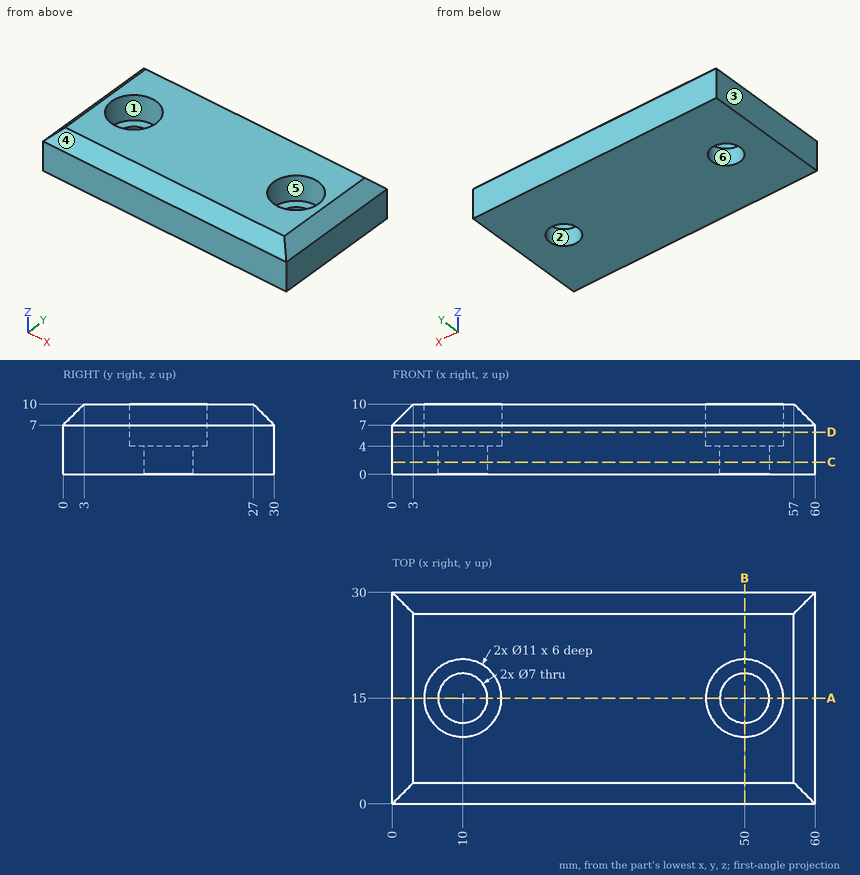
Answer from the drawing. Dimensions are ordinates in mm from the lowest x, y and z of the part. A direction names the side the tool comes from. Round coordinates to 2 decimals unless told otherwise and drop trailing zeros. Order: outer loops, then holes, each group sorted by start corner. A loop starts at its lowest first (then second) coordinate and runs counter-clockwise, first axis right, second up.
1) For the marked faces 5 and 6, determine the directions among +Z, -Z, +X, -X, +Y, -Y from which every point of the face is accessible in a straight line to the end or side of a thin tool.
2) The part is cut by section D-D on z = 6. Write down the section's boundary in (x, y), plus the area to 3 significant figures.
3) The mould has two halves that part along X. Classify the marked faces 1, 2, 3 and 4: released by +X, released by -X, zero draft, split by the parting line, or undercut.
4) Straight lines are drawn through the part: L1, parallel to Y at x = 50, z = 1.1; L2, parallel to X at y = 19, z = 7.5; L3, parallel to X at y = 20, z = 7.25. For each, find the intervals that lie inside material, in ascending order.
5) The part is cut by section B-B on x = 50. Write down the section's boundary in (y, z).
6) Flat-ended cylindrical pins translate along their axes: pin 1 (5.5 mm diameter, centred on x = 50, y = 15, fed in from +Z); pin 2 (1.5 mm diameter, centred on y = 18, z = 8.5, fed in from -X). Find the tip coordinate at first contact, or state that the pin passes through.
7) The part is cut by section A-A on y = 15. Write down the section's boundary in (x, z).
8) The part is cut by section C-C on z = 1.75. Write down the section's boundary in (x, y), plus the area to 3 significant figures.
Resolved:
1. face 5: +Z
1. face 6: +Z, -Z
2. outline: (0, 0) - (60, 0) - (60, 30) - (0, 30) - close; hole circle Ø11 at (10, 15); hole circle Ø11 at (50, 15)
2. area: 1,610 mm2
3. face 1: undercut
3. face 2: undercut
3. face 3: released by -X
3. face 4: zero draft
4. L1: y = 0 to 11.5, 18.5 to 30
4. L2: x = 0.5 to 6.23, 13.77 to 46.23, 53.77 to 59.5
4. L3: x = 0.25 to 7.71, 12.29 to 47.71, 52.29 to 59.75
5. outline: (0, 0) - (11.5, 0) - (11.5, 4) - (9.5, 4) - (9.5, 10) - (3, 10) - (0, 7) - close; (18.5, 0) - (30, 0) - (30, 7) - (27, 10) - (20.5, 10) - (20.5, 4) - (18.5, 4) - close
6. pin 1: passes through
6. pin 2: stops at x = 0.75
7. outline: (0, 0) - (6.5, 0) - (6.5, 4) - (4.5, 4) - (4.5, 10) - (3, 10) - (0, 7) - close; (13.5, 0) - (46.5, 0) - (46.5, 4) - (44.5, 4) - (44.5, 10) - (15.5, 10) - (15.5, 4) - (13.5, 4) - close; (53.5, 0) - (60, 0) - (60, 7) - (57, 10) - (55.5, 10) - (55.5, 4) - (53.5, 4) - close
8. outline: (0, 0) - (60, 0) - (60, 30) - (0, 30) - close; hole circle Ø7 at (10, 15); hole circle Ø7 at (50, 15)
8. area: 1,720 mm2
